```python
from build123d import *

# Parameters (mm, degrees)
SKETCH1_W                      = 22.86
SKETCH1_H                      = 12.7
BOSS_EXTRUDE1_DEPTH            = 5.08
F_4_40_TAPPED_HOLE1_D          = 2.2606
F_4_40_TAPPED_HOLE1_DEPTH      = 7.5946
F_4_40_TAPPED_HOLE1_TIP        = 0.679152758
SKETCH5_W                      = 6.35
SKETCH5_H                      = 10.16
CUT_EXTRUDE1_DEPTH             = 2.794
F_31_0_12_DIAMETER_HOLE1_D     = 3.048
F_31_0_12_DIAMETER_HOLE1_DEPTH = 7.5946
F_31_0_12_DIAMETER_HOLE1_TIP   = 0.915711583


with BuildPart() as part:
    # Sketch1 → Boss-Extrude1 (new body)
    with BuildSketch(Plane(origin=(0, 0, 0), x_dir=(1, 0, 0), z_dir=(0, 1, 0))):
        Rectangle(SKETCH1_W, SKETCH1_H)
    extrude(amount=BOSS_EXTRUDE1_DEPTH)

    # #4-40 Tapped Hole1
    with Locations(Plane(origin=(0, 5.08, 0), x_dir=(1, 0, 0), z_dir=(0, 1, 0))):
        with Locations((0, 3.175)):
            Hole(F_4_40_TAPPED_HOLE1_D / 2, depth=F_4_40_TAPPED_HOLE1_DEPTH)
            with Locations((0, 0, -(F_4_40_TAPPED_HOLE1_DEPTH + F_4_40_TAPPED_HOLE1_TIP / 2))):  # 118° drill point
                Cone(0, F_4_40_TAPPED_HOLE1_D / 2, F_4_40_TAPPED_HOLE1_TIP, mode=Mode.SUBTRACT)

    # Sketch5 → Cut-Extrude1 (cut)
    with BuildSketch(Plane(origin=(0, 5.08, 0), x_dir=(1, 0, 0), z_dir=(0, 1, 0))):
        with Locations((-5.08, -1.27)):
            Rectangle(SKETCH5_W, SKETCH5_H)
        with Locations((5.08, -1.27)):
            Rectangle(SKETCH5_W, SKETCH5_H)
    extrude(amount=-CUT_EXTRUDE1_DEPTH, mode=Mode.SUBTRACT)

    # #31 (0.12) Diameter Hole1
    with Locations(Plane(origin=(0, 2.286, 0), x_dir=(1, 0, 0), z_dir=(0, 1, 0))):
        with Locations((-5.08, -3.81), (5.08, -3.81)):
            Hole(F_31_0_12_DIAMETER_HOLE1_D / 2, depth=F_31_0_12_DIAMETER_HOLE1_DEPTH)
            with Locations((0, 0, -(F_31_0_12_DIAMETER_HOLE1_DEPTH + F_31_0_12_DIAMETER_HOLE1_TIP / 2))):  # 118° drill point
                Cone(0, F_31_0_12_DIAMETER_HOLE1_D / 2, F_31_0_12_DIAMETER_HOLE1_TIP, mode=Mode.SUBTRACT)


solid = part.part
```
Can you work these out from the model? Positions are in its coordinate system, mm. A direction names the side the tool comes from. Coordinates: 2 decimals unless noted, no trailing zeros. Order: outer loops, then holes, each group sorted by start corner. A loop starts at its lowest first (then second) coordinate and runs counter-clockwise, first axis right, second up.
1. If we section it at A-A (z = 3.81): Please give me the cut outline in (x, y) (3 decimals).
2. If we section it at D-D (x = 0): Please give me the cut outline in (y, z), then the cut area to 3 significant figures.
3. For faces 1 (the face through (0, 2, 6.35)), 2 (the face through (-1.905, 4, 1)), which set-ups out of +Z, -Z, +X, -X, +Y, -Y let a thin tool reach every point of the face, with its end or its side?
4. If we section it at C-C (y = 4.35): Please give me the cut outline in (x, z) (3 decimals), then the cut area to 3 significant figures.
5. I'm going to push flat-ended pins straight in: pin 1 (2.5 mm diameter, centred on x = -5.08, z = 3.81, fed in from -Y); pin 2 (4 mm diameter, centred on x = 5.08, z = 3.81, fed in from +Y); pin 3 (1.4 mm diameter, centred on x = 6.5, y = 4, fed in from +Z). Where does each tip first touch, or does it pass through?
6. Thinking about a two-plate mould opening in Z: for faces 3 (the face through (0, 3, -6.35)), 4 (the face through (-0.2, 5.08, -1.5)), 5 (the face through (-0.608, 2.504, -4.128)), which applies, +Z half, -Z half, draft (parallel to the pull), parting line (faces both ways), or undercut?
7. If we section it at B-B (x = 5.08): Please give me the cut outline in (y, z), then the cut area to 3 significant figures.
8. I need wall thicknesses on line 1 (X direction, y = 3.3, z = 1) (3 decimals); line 2 (Z direction, x = 5.08, y = 0.7); line 3 (Z direction, x = 0, y = 3.1). Which ranges of each line are inside material? Lowest first, please.
Entries:
1. outline: (-11.43, 0) - (-6.604, 0) - (-6.604, 2.286) - (-8.255, 2.286) - (-8.255, 5.08) - (-11.43, 5.08) - close; (-3.556, 0) - (3.556, 0) - (3.556, 2.286) - (1.905, 2.286) - (1.905, 5.08) - (-1.905, 5.08) - (-1.905, 2.286) - (-3.556, 2.286) - close; (6.604, 0) - (11.43, 0) - (11.43, 5.08) - (8.255, 5.08) - (8.255, 2.286) - (6.604, 2.286) - close
2. outline: (0, -6.35) - (5.08, -6.35) - (5.08, -4.31) - (0, -4.31) - close; (0, -2.04) - (5.08, -2.04) - (5.08, 6.35) - (0, 6.35) - close
2. area: 53.0 mm2
3. face 1: +Z, +X, -X, +Y, -Y
3. face 2: +Z, +Y
4. outline: (-11.43, -6.35) - (11.43, -6.35) - (11.43, 6.35) - (8.255, 6.35) - (8.255, -3.81) - (1.905, -3.81) - (1.905, 6.35) - (-1.905, 6.35) - (-1.905, -3.81) - (-8.255, -3.81) - (-8.255, 6.35) - (-11.43, 6.35) - close; hole circle Ø2.261 at (0, -3.175)
4. area: 157 mm2
5. pin 1: passes through
5. pin 2: stops at y = 2.29
5. pin 3: stops at z = -3.81
6. face 3: -Z half
6. face 4: draft
6. face 5: undercut
7. outline: (0, -6.35) - (5.08, -6.35) - (5.08, -3.81) - (2.29, -3.81) - (2.29, 2.29) - (0, 2.29) - close; (0, 5.33) - (2.29, 5.33) - (2.29, 6.35) - (0, 6.35) - close
7. area: 29.2 mm2
8. line 1: x = -11.43 to -8.255, -1.905 to 1.905, 8.255 to 11.43
8. line 2: z = -6.35 to 2.29, 5.33 to 6.35
8. line 3: z = -6.35 to -4.31, -2.04 to 6.35
